```python
from build123d import *

# Parameters (mm, degrees)
SKETCH1_R           = 1.5
BOSS_EXTRUDE1_DEPTH = 75
FILLET1_R           = 60
FILLET2_R           = 10
CUT_EXTRUDE1_DEPTH  = 4
SKETCH4_R           = 2.9
CUT_EXTRUDE2_DEPTH  = 30


with BuildPart() as part:
    # Sketch1 → Boss-Extrude1 (new body)
    with BuildSketch(Plane(origin=(0, 0, 0), x_dir=(1, 0, 0), z_dir=(0, 1, 0))):
        with BuildLine():
            Line((56.591696316, 15.21100727), (88.688017257, 15.21100727))
            ThreePointArc((88.688017257, 15.21100727), (90.560043963, 14.668289132), (91.851509041, 13.208444991))
            Line((91.851509041, 13.208444991), (99.675235919, -3.319985773))
            ThreePointArc((99.675235919, -3.319985773), (98.430900842, -29.01009942), (76.38895534, -42.264643828))
            Line((76.38895534, -42.264643828), (56.769767513, -43.264113173))
            ThreePointArc((56.769767513, -43.264113173), (55.749067562, -43.165700148), (54.80069704, -42.775691342))
            Line((54.80069704, -42.775691342), (40.459976718, -34.234343632))
            ThreePointArc((40.459976718, -34.234343632), (33.526592489, -41.048356801), (25.465280206, -46.481388792))
            Line((25.465280206, -46.481388792), (75, -44.5))
            ThreePointArc((75, -44.5), (100.341650726, -30.101348895), (100.945295539, -0.961067014))
            Line((100.945295539, -0.961067014), (77.559049402, 42.258960334))
            ThreePointArc((77.559049402, 42.258960334), (73.883135286, 46.090390077), (68.764033965, 47.5))
            Line((68.764033965, 47.5), (23.510635891, 47.5))
            ThreePointArc((23.510635891, 47.5), (43.938112979, 35.337799568), (56.591696316, 15.21100727))
        make_face()
        with Locations(Location((71.835494757, 42.654234046, 0), (0, 0, 270))):
            Circle(SKETCH1_R, mode=Mode.SUBTRACT)
        with Locations(Location((40.293422434, -41.885064382, 0), (0, 0, 270))):
            Circle(SKETCH1_R, mode=Mode.SUBTRACT)
        with Locations(Location((42.137334928, 43.5, 0), (0, 0, 270))):
            Circle(SKETCH1_R, mode=Mode.SUBTRACT)
        with Locations(Location((83.354686129, 23.142870245, 0), (0, 0, 270))):
            Circle(SKETCH1_R, mode=Mode.SUBTRACT)
    extrude(amount=BOSS_EXTRUDE1_DEPTH)

    # Fillet1
    fillet1_edges = [part.edges().sort_by_distance(p)[0] for p in [
        (56.591696316, 37.5, -15.21100727),
    ]]
    fillet(fillet1_edges, radius=FILLET1_R)

    # Fillet2
    fillet2_edges = [part.edges().sort_by_distance(p)[0] for p in [
        (40.459976718, 37.5, 34.234343632),
    ]]
    fillet(fillet2_edges, radius=FILLET2_R)

    # Sketch3 → Cut-Extrude1 (cut)
    with BuildSketch(Plane(origin=(0, 72, 0), x_dir=(1, 0, 0), z_dir=(0, 1, 0))):
        with BuildLine():
            Line((39.137334928, 43.5), (39.137334928, 48.914062906))
            Line((39.137334928, 48.914062906), (45.137334928, 48.914062906))
            Line((45.137334928, 48.914062906), (45.137334928, 43.5))
            ThreePointArc((45.137334928, 43.5), (42.137334928, 40.5), (39.137334928, 43.5))
        make_face()
        with BuildLine():
            Line((74.41261178, 41.11850365), (77.272251707, 45.917280019))
            Line((77.272251707, 45.917280019), (72.118017661, 48.988740812))
            Line((72.118017661, 48.988740812), (69.258377734, 44.189964442))
            ThreePointArc((69.258377734, 44.189964442), (70.299764361, 40.077117023), (74.41261178, 41.11850365))
        make_face()
        with BuildLine():
            Line((81.936736501, 25.786621151), (87.421531644, 28.728336732))
            Line((87.421531644, 28.728336732), (90.2574309, 23.44083492))
            Line((90.2574309, 23.44083492), (84.772635757, 20.499119339))
            ThreePointArc((84.772635757, 20.499119339), (80.710935223, 21.724920617), (81.936736501, 25.786621151))
        make_face()
        with BuildLine():
            Line((37.298688778, -42.062744804), (37.612282879, -47.348250065))
            Line((37.612282879, -47.348250065), (43.60175019, -46.99288922))
            Line((43.60175019, -46.99288922), (43.288156089, -41.707383959))
            ThreePointArc((43.288156089, -41.707383959), (40.115742012, -38.890330726), (37.298688778, -42.062744804))
        make_face()
    cut_extrude1 = extrude(amount=-CUT_EXTRUDE1_DEPTH, mode=Mode.SUBTRACT)

    # Mirror1: Cut-Extrude1 across plane
    add(cut_extrude1.mirror(Plane.ZX.offset(37.5)), mode=Mode.SUBTRACT)

    # Sketch4 → Cut-Extrude2 (cut)
    with BuildSketch(Plane(origin=(0, 0, -47.5), x_dir=(-1, 0, 0), z_dir=(0, 0, -1))):
        with Locations((-61.510635891, 57.5)):
            Circle(SKETCH4_R)
        with Locations((-36.510635891, 57.5)):
            Circle(SKETCH4_R)
        with Locations((-36.510635891, 17.5)):
            Circle(SKETCH4_R)
        with Locations((-61.510635891, 17.5)):
            Circle(SKETCH4_R)
    extrude(amount=-CUT_EXTRUDE2_DEPTH, mode=Mode.SUBTRACT)


solid = part.part
```
Source: CAD feature listing. Evaluate the final solid. Frame: model axes, mm. A direction names the side the tool comes from. Give positions to 0.01 mm unless a question says otherwise; leave off trailing zeros. Loops run counter-clockwise (first coordinate to the right, second up) from the corner with the lowest first, then second, coordinate; pieces in that order, holes last. Notation, with made-up numbers: (75, -16.75) -> (130, -16.75) arc R25 ccw to (130, 15.25) -> close; hole circle Ø4 at (-9, 1.25). An arc over 180 degrees is marked (long way). Use a Markdown table: item, result. Add a question column.
(1) Access query for faces 1 (the face through (39.137, 70, -45)), 2 (the face through (84, 72, -25)), 3 (the face through (30.72, 36.98, 43.19)). Directions: +Z, -Z, +X, -X, +Y, -Y. A direction counts if a zero-diameter tool reaches every point of the face in a straight line with its end or side. Return the directions, or none.
(2) Section query B-B (y = 57.5). Count the separate pieces of the cut face and the enclosed holes in it, then the cut area to 3 significant figures.
(3) Ray query, line 1 (Y direction, x = 69.5, z = -41); line 2 (X direction, y = 57.5, z = -45.5); line 3 (X direction, y = 17, z = -43). Return the intervals inside material, ascending.
(4) First-contact query: pin 1 Ø6 at (x, z) = (73, -42.5) entering from +Y; pin 2 Ø4.5 at (x, y) = (61.51, 17.5) entering from -Z; pin 3 Ø5 at (y, z) = (60, 13.5) entering from +X; pin 4 Ø5 at (y, z) = (19.5, 19.5) entering from -X. Flat tips, straight axial feed; report the tip coordinate or a pass-through.
(5) Section query C-C (z = 9). Output: boundary loops of the cut face in (x, y).
(6) Pull-direction query (X, two-part tool) for faces 4 (the face through (35.134, 36.975, -42.214)), 5 (the face through (70.243, 70.028, -40.112)), 6 (the face through (40, 68, 44)), 7 (the face through (49.886, 36.975, 45.505)); classes: +X half, -X half, draft (parallel to the pull), parting line (faces both ways), or undercut.
(7) Section query A-A (x = 97.5). Output: boundary loops of the cut face in (y, z).
Checked values:
| question | item | result |
|---|---|---|
| 1 | face 1 | -Z |
| 1 | face 2 | none |
| 1 | face 3 | -X, +Y, -Y |
| 2 | separate pieces | 3 |
| 2 | enclosed holes | 4 |
| 2 | area | 1,250 mm^2 |
| 3 | line 1 | 0 to 3, 7 to 68, 72 to 75 |
| 3 | line 2 | 28.87 to 33.61, 39.41 to 58.61, 64.41 to 74.76 |
| 3 | line 3 | 39.37 to 40.72, 43.55 to 58.65, 64.37 to 70.38, 73.3 to 77.12 |
| 4 | pin 1 | y = 75 |
| 4 | pin 2 | z = 42.91 |
| 4 | pin 3 | x = 104.5 |
| 4 | pin 4 | x = 101.39 |
| 5 | outline | (101.63, 0) -> (103.88, 0) -> (103.88, 75) -> (101.63, 75) -> close |
| 6 | face 4 | -X half |
| 6 | face 5 | undercut |
| 6 | face 6 | undercut |
| 6 | face 7 | +X half |
| 7 | outline | (0, -5.41) -> (75, -5.41) -> (75, -1.28) -> (0, -1.28) -> close; (0, 30.46) -> (75, 30.46) -> (75, 34.08) -> (0, 34.08) -> close |
